```python
from build123d import *

# Parameters (mm, degrees)
F1_DEPTH = 9.525
F2_COUNT = 7
F3_R     = 15.24
F4_DEPTH = 9.525
F5_R     = 4
F6_DEPTH = 9.526


with BuildPart() as f1:
    # F0 (on Front) → F1 (new body)
    with BuildSketch(Plane.XZ):
        with BuildLine():
            ThreePointArc((-5.2396074411, 14.3109787878), (-0.9038291333, 15.2131749776), (3.5082727862, 14.8306986369))
            ThreePointArc((3.5082727862, 14.8306986369), (2.9205603088, 16.9463674955), (2.0085985954, 18.9438124907))
            ThreePointArc((2.0085985954, 18.9438124907), (-1.1297864166, 19.0164687219), (-4.2374916987, 18.5727263509))
            ThreePointArc((-4.2374916987, 18.5727263509), (-4.9065328108, 16.4813524805), (-5.2396074411, 14.3109787878))
        make_face()
    extrude(amount=F1_DEPTH)


with BuildPart() as f2_1:
    # F2: instance of F1
    add(f1.part.rotate(Axis((0, 0, 0), (0, -1, 0)), 1 * 360 / F2_COUNT))


with BuildPart() as f2_2:
    # F2: instance of F1
    add(f1.part.rotate(Axis((0, 0, 0), (0, -1, 0)), 2 * 360 / F2_COUNT))


with BuildPart() as f2_3:
    # F2: instance of F1
    add(f1.part.rotate(Axis((0, 0, 0), (0, -1, 0)), 3 * 360 / F2_COUNT))


with BuildPart() as f2_4:
    # F2: instance of F1
    add(f1.part.rotate(Axis((0, 0, 0), (0, -1, 0)), 4 * 360 / F2_COUNT))


with BuildPart() as f2_5:
    # F2: instance of F1
    add(f1.part.rotate(Axis((0, 0, 0), (0, -1, 0)), 5 * 360 / F2_COUNT))


with BuildPart() as f2_6:
    # F2: instance of F1
    add(f1.part.rotate(Axis((0, 0, 0), (0, -1, 0)), 6 * 360 / F2_COUNT))


with BuildPart() as f1_1:
    add(f1.part)

    add(f2_1.part)  # F4 merges F2_1

    add(f2_2.part)  # F4 merges F2_2

    add(f2_3.part)  # F4 merges F2_3

    add(f2_4.part)  # F4 merges F2_4

    add(f2_5.part)  # F4 merges F2_5

    add(f2_6.part)  # F4 merges F2_6
    # F3 (on Front) → F4 (join, through all)
    with BuildSketch(Plane.XZ):
        Circle(F3_R)
    extrude(amount=F4_DEPTH)

    # F5 (on face) → F6 (cut, through all)
    with BuildSketch(Plane.XZ.offset(9.525)):
        Circle(F5_R)
    extrude(amount=-F6_DEPTH, mode=Mode.SUBTRACT)


solid = f1_1.part
```
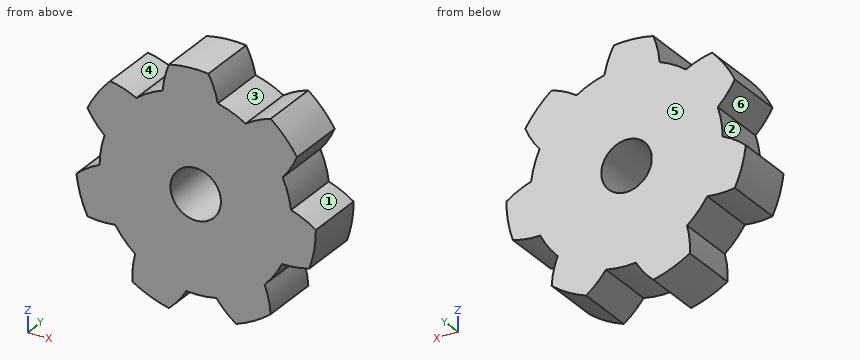
Source: CAD feature listing. Evaluate the final solid. Frame: model axes, mm. Face numbers are marked on the shaded views. A direction names the side the tool comes from. Coordinates: 2 decimals unless noted, no trailing zeros. Order: outer loops, then holes, each group sorted by start corner. A loop starts at its lowest first (then second) coordinate and runs counter-clockwise, first axis right, second up. Notation, with made-up numbers: (16.5, 52.25) - (33.5, 52.25) arc R15 cw to (33.5, 63.25) - close; hole circle Ø10 at (56.5, 12.25). An arc over 180 degrees is marked (long way). One line per item, written item: value.
1) Cut plane C-C on z = 16.5. Output: boundary loops of the cut face in (x, y) (3 decimals).
Computed values:
outline: (-4.902, -9.525) - (3.075, -9.525) - (3.075, 0) - (-4.902, 0) - close
2) Ray query, line 1 (Z direction, x = 0, y = -5.25); line 2 (X direction, y = -2.25, z = -16); line 3 (X direction, y = -7.25, z = 2.5). Return the intervals inside material, ascending. Write a range as [from, to].
Computed values:
line 1: z = [-15.24, -4], [4, 19.05]
line 2: x = [-10.04, -2.01], [4.2, 10.34]
line 3: x = [-15.03, -3.12], [3.12, 15.03]
3) Mould query, pull axis X, two halves, no side actions, for the marked faces 4, 5 and 6. Classes: released by +X, released by -X, zero draft, split by the parting line, or undercut.
Computed values:
face 4: undercut
face 5: zero draft
face 6: released by -X
4) Cut plane D-D on z = -12.5. Output: boundary loops of the cut face in (x, y) (3 decimals).
Computed values:
outline: (-9.752, -9.525) - (11.521, -9.525) - (11.521, 0) - (-9.752, 0) - close
5) Contact query for flat-ended pins moving along their axis: pin 1 (5 mm diameter, centred on y = -6, z = 7, fed in from -X); pin 2 (1.5 mm diameter, centred on y = -4.5, z = -2.5, fed in from +X). Output: stop coordinate, or through.
Computed values:
pin 1: stops at x = -17.16
pin 2: stops at x = 18.97
6) Cut plane A-A on x = 0. Output: boundary loops of the cut face in (y, z) (3 decimals), plus the area to 3 significant figures.
Computed values:
outline: (-9.525, -15.24) - (0, -15.24) - (0, -4) - (-9.525, -4) - close; (-9.525, 4) - (0, 4) - (0, 19.05) - (-9.525, 19.05) - close
area: 250 mm^2
7) Reachability of the marked faces 1, 2 and 3 from +Z, -Z, +X, -X, +Y, -Y: full face, straight path, thin tool, end or side. Return the list, or none.
Computed values:
face 1: +X, +Y, -Y
face 2: -X, +Y, -Y
face 3: +Z, +Y, -Y
